Build history of the part. All positions in model axes, mm. A direction names the side the tool comes from. Coordinates: 2 decimals unless noted, no trailing zeros. Loops run counter-clockwise (first coordinate to the right, second up) from the corner with the lowest first, then second, coordinate; pieces in that order, holes last.
(1) Flat gauge pins, fed straight in: P1, Ø1.6, axis at y = -17, z = -54.5, coming from the +X side; P2, Ø3, axis at y = -13.5, z = -7.5, coming from the +X side; P3, Ø1.5, axis at x = -27.5, y = -14.5, coming from the +Z side; P4, Ø12, axis at x = -25, z = 5, coming from the -Y side. Where does each tip first touch, or does it go through?
(2) Slice it at C-C (x = -17). Give the cut face in (y, z).
(3) Slice it at D-D (z = 7). Give the cut face in (x, y).
(4) Two-plate mould, pull along Z, no slides. Class faces 1 (the face through (20.804, -13, -52)), 2 (the face through (7.511, -12.522, -27.626)), 3 (the face through (-9.811, -13, -17)), 4 (the face through (-27, -13, 22.368)): pulls with the +Z half, pulls with the -Z half, needs draft (parallel to the pull), parting line crosses it, or undercut.
(5) Wall check: L1, parallel to X at y = -17.5, z = -55; L2, parallel to X at y = -22, z = -44; L3, parallel to X at y = -16, z = -23.5. Give the ranges that are in metal, low to high.
(6) Slice it at A-A (z = -46). Give the cut face in (x, y), and give its area (3 significant figures).
(7) Slice it at B-B (z = -34). Give the cut face in (x, y), and give its area (3 significant figures).
(8) Tool access for faces 5 (the face through (13.617, -12.522, -47.6)), 6 (the face through (-2.94, -12.52, 0.78)), 7 (the face through (0.249, -12.522, -50.912)): list every direction of +Z, -Z, +X, -X, +Y, -Y with a clear straight run to the whole face (end or side of a thin tool).
from build123d import *

# Parameters (mm, degrees)
F1_DEPTH = 25.4


with BuildPart() as f1:
    # F0 (on Front) → F1 (new body)
    with BuildSketch(Plane.XZ):
        Polygon((-4.807071, 1.577358), (-18.804783, 19.995399), (-19.201438, 20.510813), (-18.328309, 22.415822), (-19.470988, 22.93955), (-20.851724, 22.225376), (-21.888541, 23.302863), (-22.851409, 22.844328), (-23.918144, 25.084342), (-23.217195, 26.69334), (-24.327368, 27.17698), (-26.422277, 22.368211), (-28.279129, 22.368211), (-28.883137, 21.677395), (-32.133359, 17.464144), (-33.818658, 15.598277), (-34.480739, 14.755626), (-34.480739, 12.769381), (-33.818658, 13.371274), (-31.772222, 13.371274), (-30.989761, 14.033356), (-29.725786, 14.940684), (-26.475566, 14.940684), (-23.919655, 14.940684), (-23.405911, 15.598277), (-21.479854, 14.093545), (-20.130018, 11.494951), (-15.262124, 1.325255), (-12.446605, -3.467118), (-8.432992, -9.51749), (-7.893849, -12.752342), (-9.810799, -15.927291), (-9.810799, -18.563095), (-8.383603, -20.670711), (-6.653502, -22.416285), (0, -25.213145), (4.167965, -26.388429), (6.779463, -26.259693), (8.263807, -29.03047), (10.698803, -30.795518), (13.631921, -36.270678), (12.499449, -44.314019), (10.698803, -48.52825), (8.607689, -56.42225), (8.717785, -58.655619), (11.401466, -56.10612), (10.698803, -55.366475), (11.870418, -51.878039), (15.41289, -43.200385), (16.533865, -24.944445), (20.064365, -42.185199), (20.804008, -49.071185), (20.804008, -52.51319), (20.804008, -55.267211), (19.592239, -58.638137), (19.239724, -60.599003), (21.46933, -59.010107), (22.771196, -56.008819), (22.771196, -49.071185), (22.338118, -40.285911), (23.370066, -36.270678), (20.118674, -30.201407), (20.118674, -27.645931), (20.118674, -20.128688), (27.467125, -37.082013), (27.467125, -39.04331), (28.99437, -41.676154), (28.832508, -40.571583), (29.336633, -40.497709), (30.216336, -41.676154), (29.67385, -37.97416), (30.246906, -37.401102), (31.513076, -40.497709), (31.012544, -37.082013), (29.280987, -36.023837), (27.111409, -29.904326), (26.01208, -27.055074), (22.192179, -18.312787), (21.46933, -16.963469), (18.276872, -13.64822), (15.57556, -10.701334), (7.717195, -7.508874), (5.507031, -6.035431), (2.928506, -3.456905), (-1.123464, 0), align=None)
        Polygon((0, -25.213145), (-6.653502, -22.416285), (-7.403816, -29.544273), (-9.385442, -37.977327), (-8.536174, -40.962219), (-7.403816, -42.094577), (-3.761253, -48.406478), (-1.043809, -53.469059), (1.077536, -57.421111), (1.354785, -57.54178), (1.354785, -58.036473), (2.10664, -58.543845), (3.545563, -54.87987), (2.500879, -54.4696), (-2.067813, -47.252391), (-3.49469, -44.776939), (-5.039291, -40.263818), (-2.894435, -32.09877), align=None)
        Polygon((-0.742696, -37.977327), (0, -25.213145), (-2.894435, -32.09877), (-3.369526, -40.263818), (-3.49469, -41.377133), (-3.49469, -44.776939), (-2.067813, -47.252391), (-1.458444, -44.776939), align=None)
        Polygon((-1.043809, -53.469059), (-3.761253, -48.406478), (-4.477841, -55.21406), (-5.608209, -57.388235), (-1.396718, -56.248265), (-1.348698, -55.792075), (-1.348698, -53.771246), align=None)
    extrude(amount=F1_DEPTH)


solid = f1.part
Response values:
1. P1: stops at x = 22.77
1. P2: stops at x = 11.39
1. P3: stops at z = 22.37
1. P4: passes through
2. outline: (-25.4, 4.96) - (0, 4.96) - (0, 17.62) - (-25.4, 17.62) - close
3. outline: (-17.98, -25.4) - (-8.93, -25.4) - (-8.93, 0) - (-17.98, 0) - close
4. face 1: undercut
4. face 2: pulls with the -Z half
4. face 3: needs draft
4. face 4: pulls with the +Z half
5. L1: x = -4.46 to -1.35, -0.22 to 3.5, 8.98 to 10.82, 20.8 to 22.77
5. L2: x = -6.3 to -3.76, -3.49 to -1.38, 12.54 to 15.09, 20.26 to 22.52
5. L3: x = -6.77 to 20.12, 21.58 to 24.46
6. outline: (-5.15, -25.4) - (-1.76, -25.4) - (-1.76, 0) - (-5.15, 0) - close; (11.78, -25.4) - (14.27, -25.4) - (14.27, 0) - (11.78, 0) - close; (20.47, -25.4) - (22.62, -25.4) - (22.62, 0) - (20.47, 0) - close
6. area: 204 mm2
7. outline: (-8.45, -25.4) - (-3.39, -25.4) - (-3.39, 0) - (-8.45, 0) - close; (-3.01, -25.4) - (-0.51, -25.4) - (-0.51, 0) - (-3.01, 0) - close; (12.42, -25.4) - (15.98, -25.4) - (15.98, 0) - (12.42, 0) - close; (18.39, -25.4) - (22.15, -25.4) - (22.15, 0) - (18.39, 0) - close; (26.13, -25.4) - (28.56, -25.4) - (28.56, 0) - (26.13, 0) - close
7. area: 440 mm2
8. face 5: -Z, +Y, -Y
8. face 6: +Z, +X, +Y, -Y
8. face 7: +Y, -Y
